Can you work these out from the model? Positions are in its coordinate system, mm. A direction names the side the tool comes from. Coordinates: 2 decimals unless noted, no trailing zeros. Order: outer loops, then holes, each group sorted by start corner. A loop starts at its lowest first (then second) coordinate and runs counter-clockwise, first axis right, second up.
Autodesk Inventor part; units mm, degrees
ref_plane "YZ Plane" through (0, 0, 0) normal (1, 0, 0) x (0, 1, 0)
ref_plane "XZ Plane" through (0, 0, 0) normal (0, 1, 0) x (-1, 0, 0)
ref_plane "XY Plane" through (0, 0, 0) normal (0, 0, 1) x (1, 0, 0)
sketch "Sketch1" plane through (0, 0, 0) normal (0, 0, 1) x (1, 0, 0)
  line L0 (-27.5, -27.5) -> (27.5, -27.5)
  line L1 (27.5, -27.5) -> (27.5, 27.5)
  line L2 (27.5, 27.5) -> (-27.5, 27.5)
  line L3 (-27.5, 27.5) -> (-27.5, -27.5)
  line L4 (-27.5, -27.5) -> (27.5, 27.5) construction
  line L5 (27.5, -27.5) -> (-27.5, 27.5) construction
  line L6 (-20, 14.15) -> (20, 14.15) construction
  line L7 (20, 14.15) -> (20, -14.15) construction
  line L8 (20, -14.15) -> (-20, -14.15) construction
  line L9 (-20, -14.15) -> (-20, 14.15) construction
  line L10 (-20, 14.15) -> (20, -14.15) construction
  line L11 (20, 14.15) -> (-20, -14.15) construction
  line L12 (0, -27.5) -> (0, 27.5) construction
  line L13 (-27.5, 0) -> (27.5, 0)
  line L14 (17, 11.25) -> (-17, 11.25) construction
  line L15 (-17, 11.25) -> (-17, -11.25) construction
  line L16 (-17, -11.25) -> (17, -11.25) construction
  line L17 (17, -11.25) -> (17, 11.25) construction
  line L18 (17, 11.25) -> (-17, -11.25) construction
  line L19 (-17, 11.25) -> (17, -11.25) construction
  line L20 (20.25, -12.4) -> (20.25, 12.4)
  line L21 (-18.5, -27.5) -> (-18.5, -30.5)
  line L22 (-18.5, -30.5) -> (18.5, -30.5)
  line L23 (18.5, -30.5) -> (18.5, -27.5)
  arc A0 (-18.5, -27.5) -> (-21.5, -27.5) centre (-20, -27.5) ccw
  line L24 (-24.5, -27.5) -> (-24.5, -21.5) construction
  arc A1 (21.5, -27.5) -> (18.5, -27.5) centre (20, -27.5) ccw
  line L25 (24.5, -27.5) -> (24.5, -21.5) construction
  line L26 (-18.5, 27.5) -> (-18.5, 30.5)
  line L27 (-18.5, 30.5) -> (18.5, 30.5)
  line L28 (18.5, 30.5) -> (18.5, 27.5)
  arc A2 (-21.5, 27.5) -> (-18.5, 27.5) centre (-20, 27.5) ccw
  line L29 (-24.5, 27.5) -> (-24.5, 21.5) construction
  arc A3 (18.5, 27.5) -> (21.5, 27.5) centre (20, 27.5) ccw
  line L30 (24.5, 27.5) -> (24.5, 21.5) construction
  line L31 (-12, -14.4) -> (18.25, -14.4)
  line L32 (-14, -12.4) -> (-14, -11.25)
  line L33 (-18.25, -8.25) -> (-17, -8.25)
  line L34 (-20.25, -6.25) -> (-20.25, 6.25)
  arc A4 (-14, -11.25) -> (-17, -8.25) centre (-17, -11.25) ccw
  line L35 (-12, 14.4) -> (18.25, 14.4)
  line L36 (-14, 12.4) -> (-14, 11.25)
  line L37 (-18.25, 8.25) -> (-17, 8.25)
  arc A5 (-17, 8.25) -> (-14, 11.25) centre (-17, 11.25) ccw
  arc A6 (-20.25, -6.25) -> (-18.25, -8.25) centre (-18.25, -6.25) ccw
  arc A7 (-14, -12.4) -> (-12, -14.4) centre (-12, -12.4) ccw
  arc A8 (18.25, -14.4) -> (20.25, -12.4) centre (18.25, -12.4) ccw
  arc A9 (20.25, 12.4) -> (18.25, 14.4) centre (18.25, 12.4) ccw
  arc A10 (-12, 14.4) -> (-14, 12.4) centre (-12, 12.4) ccw
  arc A11 (-18.25, 8.25) -> (-20.25, 6.25) centre (-18.25, 6.25) ccw
  line L38 (24.5, 22.25) -> (-24.5, 22.25) construction
  line L39 (-24.5, 22.25) -> (-24.5, -22.25) construction
  line L40 (-24.5, -22.25) -> (24.5, -22.25) construction
  line L41 (24.5, -22.25) -> (24.5, 22.25) construction
  line L42 (24.5, 22.25) -> (-24.5, -22.25) construction
  line L43 (-24.5, 22.25) -> (24.5, -22.25) construction
  line L44 (32.5, 26.5) -> (-32.5, 26.5) construction
  line L45 (-32.5, 26.5) -> (-32.5, -26.5) construction
  line L46 (-32.5, -26.5) -> (32.5, -26.5) construction
  line L47 (32.5, -26.5) -> (32.5, 26.5) construction
  line L48 (32.5, 26.5) -> (-32.5, -26.5) construction
  line L49 (-32.5, 26.5) -> (32.5, -26.5) construction
  circle A12 centre (-24.5, -22.25) radius 1.5 construction
  point P0 (0, 0)
  point P1 (21.5, 27.5)
  point P2 (-21.5, 27.5)
  point P3 (21.5, -27.5)
  point P4 (20.25, 0)
  point P5 (-14, -14.4)
  point P6 (20.25, -14.4)
  point P7 (-20.25, -8.25)
  point P8 (-14, 14.4)
  point P9 (20.25, 14.4)
  point P10 (-20.25, 8.25)
  point P11 (-20.25, 0)
  dimension "d0" = 55
  dimension "d1" = 55
  dimension "d2" = 40
  dimension "d3" = 28.3
  dimension "d4" = 34
  dimension "d5" = 22.5
  dimension "d8" = 1.5
  dimension "d9" = 6
  dimension "d10" = 6
  dimension "d11" = 3
  dimension "d35" = 6
  dimension "d36" = 0.25
  dimension "d37" = 0.25
  dimension "d38" = 2
  dimension "d39" = 6
  dimension "d40" = 8.5
  dimension "d41" = 16
  dimension "d42" = 1
  dimension "d43" = 3
  dimension "d44" = 3.75
  dimension "d45" = 49
extrude "Extrusion1" add sketch "Sketch1" along normal blind 5 contours L3 L13 L34 A6 L33 A4 L32 A7 L31 A8 L20 L1 L0 A1 A0 | L0 L23 L22 L21
hole "M3" at (-17, -11.25, 0) at (-24.5, -22.25, 0) at (24.5, -22.25, 0) direction (0, 0, 1) diameter 2.459 end through all
chamfer "C0.5" distance 0.5 angle 45 2 edges at (-18.5, -30.5, 2.5) (18.5, -30.5, 2.5)
sketch "Sketch3" plane through (-18, -30.5, 0) normal (0, -1, 0) x (1, 0, 0)
  line L0 (18, 0) -> (18, 5)
  line L1 (0, 5) -> (36, 5)
  point P0 (18, 2.5)
sketch "Sketch2" plane through (21.5, -27.5, 0) normal (0, -1, 0) x (1, 0, 0)
  line L0 (3, 0) -> (3, 5)
  line L1 (-49, 5) -> (6, 5)
  line L2 (-46, 0) -> (-46, 5)
  line L3 (-49, 5) -> (6, 5)
  line L4 (0, 0) -> (6, 0)
  line L5 (-49, 0) -> (-43, 0)
  point P0 (0, 5)
  point P1 (-43, 5)
  point P2 (-46, 2.5)
  point P3 (3, 2.5)
  point P4 (3, 0)
  point P5 (3, 0)
  point P6 (3, 0)
hole "Side-M2-6(1)" at (24.5, -27.5, 2.5) at (-24.5, -27.5, 2.5) direction (0, 1, 0) diameter 1.567 depth 6
hole "Side-M2-6(2)" at (0, -30.5, 2.5) direction (0, 1, 0) diameter 1.567 depth 6
mirror "Mirror1" about plane through (0, 0, 0) normal (0, 1, 0)
equation "\"d37\" = d36"
equation "\"d26\" = d9"
properties part number "HeadUpperFrame" material "Acetal Resin, Black"
1. Imagine slicing it at A-A on x = 0. Please give me the cut outline in (y, z).
Completed:
outline: (-30.5, 0) - (-14.4, 0) - (-14.4, 5) - (-30.5, 5) - (-30.5, 3.28) - (-24.5, 3.28) - (-24.5, 1.72) - (-30.5, 1.72) - close; (14.4, 0) - (30.5, 0) - (30.5, 1.72) - (24.5, 1.72) - (24.5, 3.28) - (30.5, 3.28) - (30.5, 5) - (14.4, 5) - close
2. Imagine slicing it at B-B on z = 2.5. Give the number of separate pieces and of enclosed holes in the cut face, then the cut area to 3 significant figures.
Completed:
separate pieces: 1
enclosed holes: 3
area: 2,070 mm2
3. On a 3-axis mill with a long thin cutter (end or side, diameter ignored), from which of +Z, -Z, +X, -X, +Y, -Y can I reach the whole of each face in a straight line? I mean faces 4 (the cylindrical face through (-13.43, 13.8, 2.46)), 5 (the cylindrical face through (-24.534, -25.319, 3.283)), 6 (the flat face through (-24, 27.5, 1)). Say none if no direction works.
Completed:
face 4: +Z, -Z
face 5: -Y
face 6: +Z, -Z, -X, +Y
4. Please list where these lines run through material, in increasing order: probe 1 along X at (y, z) = (-22.25, 3.25); probe 2 along Y at (x, z) = (-17, 2.1); probe 3 along X at (y, z) = (24.15, 2.5).
Completed:
probe 1: x = -27.5 to -25.73, -23.27 to 23.27, 25.73 to 27.5
probe 2: y = -30.5 to -12.48, -10.02 to -8.25, 8.25 to 10.02, 12.48 to 30.5
probe 3: x = -27.5 to -25.28, -23.72 to 23.72, 25.28 to 27.5
5. I'm going to push flat-ended pins straight in: pin 1 (1.4 mm diameter, centred on x = 0, z = 2.5, fed in from +Y); pin 2 (2.5 mm diameter, centred on x = -25.5, z = 2.5, fed in from +Y); pin 3 (2 mm diameter, centred on x = -17, y = 11.25, fed in from -Z); pin 4 (2.5 mm diameter, centred on x = -24.5, z = 3.5, fed in from -Y). Where does each tip first touch, or does it pass through?
Completed:
pin 1: stops at y = 24.5
pin 2: stops at y = 27.5
pin 3: passes through
pin 4: stops at y = -27.5
6. Thinking about a two-plate mould opening in X: for faces 1 (the flat face through (0, -30.5, 1)), 2 (the flat face through (3, 14.4, 2)), 3 (the flat face through (-27.5, 0, 2)), which applies, pulls with the +X half, pulls with the -X half, needs draft (parallel to the pull), parting line crosses it, or undercut?
Completed:
face 1: needs draft
face 2: undercut
face 3: pulls with the -X half
